```python
from build123d import *

# Parameters (mm, degrees)
SKETCH1_W                                      = 65
SKETCH1_H                                      = 40
BOSS_EXTRUDE1_DEPTH                            = 7.5
F_4_40_TAPPED_HOLE1_D                          = 2.2606
F_4_40_TAPPED_HOLE1_DEPTH                      = 7.6
F_4_40_TAPPED_HOLE1_TIP                        = 0.679152758
F_4_40_TAPPED_HOLE2_D                          = 2.2606
F_4_40_TAPPED_HOLE2_DEPTH                      = 7.6
F_4_40_TAPPED_HOLE2_TIP                        = 0.679152758
CBORE_FOR_4_SOCKET_HEAD_CAP_SCREW1_D           = 3.2639
CBORE_FOR_4_SOCKET_HEAD_CAP_SCREW1_CBORE_D     = 5.55752
CBORE_FOR_4_SOCKET_HEAD_CAP_SCREW1_CBORE_DEPTH = 2.8448


with BuildPart() as part:
    # Sketch1 → Boss-Extrude1 (new body)
    with BuildSketch(Plane(origin=(0, 0, 0), x_dir=(1, 0, 0), z_dir=(0, 1, 0))):
        Rectangle(SKETCH1_W, SKETCH1_H)
    extrude(amount=BOSS_EXTRUDE1_DEPTH)

    # #4-40 Tapped Hole1
    with Locations(Plane.XY.offset(20)):
        with Locations((-15, 3.75), (15, 3.75)):
            Hole(F_4_40_TAPPED_HOLE1_D / 2, depth=F_4_40_TAPPED_HOLE1_DEPTH)
            with Locations((0, 0, -(F_4_40_TAPPED_HOLE1_DEPTH + F_4_40_TAPPED_HOLE1_TIP / 2))):  # 118° drill point
                Cone(0, F_4_40_TAPPED_HOLE1_D / 2, F_4_40_TAPPED_HOLE1_TIP, mode=Mode.SUBTRACT)

    # #4-40 Tapped Hole2
    with Locations(Plane(origin=(0, 0, -20), x_dir=(-1, 0, 0), z_dir=(0, 0, -1))):
        with Locations((-15, 3.75), (15, 3.75)):
            Hole(F_4_40_TAPPED_HOLE2_D / 2, depth=F_4_40_TAPPED_HOLE2_DEPTH)
            with Locations((0, 0, -(F_4_40_TAPPED_HOLE2_DEPTH + F_4_40_TAPPED_HOLE2_TIP / 2))):  # 118° drill point
                Cone(0, F_4_40_TAPPED_HOLE2_D / 2, F_4_40_TAPPED_HOLE2_TIP, mode=Mode.SUBTRACT)

    # CBORE for #4 Socket Head Cap Screw1 (through all)
    with Locations(Plane(origin=(0, 0, 0), x_dir=(-1, 0, 0), z_dir=(0, -1, 0))):
        with Locations((-28.75, -10), (-28.75, 10), (28.75, 10), (28.75, -10)):
            CounterBoreHole(CBORE_FOR_4_SOCKET_HEAD_CAP_SCREW1_D / 2, CBORE_FOR_4_SOCKET_HEAD_CAP_SCREW1_CBORE_D / 2, CBORE_FOR_4_SOCKET_HEAD_CAP_SCREW1_CBORE_DEPTH)


solid = part.part
```
Read the model definition and answer for the solid it produces. Units are mm, in the model's axes. A direction names the side the tool comes from. Give positions to 0.01 mm unless a question says otherwise; leave off trailing zeros. Order: outer loops, then holes, each group sorted by start corner. A loop starts at its lowest first (then second) coordinate and runs counter-clockwise, first axis right, second up.
(1) For faces 4 (the flat face through (-31, 2.845, -10)), 5 (the cylindrical face through (14.103, 3.062, -16.147)), 6 (the cylindrical face through (-14.103, 3.062, 16.147)), determine the directions among +Z, -Z, +X, -X, +Y, -Y from which every point of the face is accessible in a straight line to the end or side of a thin tool.
(2) For a pull along X with two mould halves and no side action, classify faces 1 (the flat face through (0, 7.5, 0)), 2 (the flat face through (26.9, 2.845, 10)), 3 (the flat face through (32.5, 4, 0)) as released by +X, released by -X, zero draft, split by the parting line, or undercut.
(3) Given pin 1 (4.5 mm diameter, centred on x = 28.5, z = -10, fed in from -Y); pin 2 (1.8 mm diameter, centred on x = -15, y = 3.75, fed in from -Z), each flat-ended and moving along its own axis, determine where each tip first touches the part or whether it passes through.
(4) Find section C-C (z = -16.5). Give the vertices of the cut face in (x, y).
(5) Find section B-B (z = -10). Give the vertices of the cut face in (x, y).
(6) Straight lines are drawn through the part: L1, parallel to Z at x = 28.75, y = 4.05; L2, parallel to X at y = 5, z = -10; L3, parallel to X at y = 3.75, z = 16.75. For each, find the intervals that lie inside material, in ascending order.
(7) Find section A-A (x = -28.75). Give the vertices of the cut face in (y, z).
Result sheet:
1. face 4: -Y
1. face 5: -Z
1. face 6: +Z
2. face 1: zero draft
2. face 2: undercut
2. face 3: released by +X
3. pin 1: stops at y = 2.84
3. pin 2: stops at z = -12.26
4. outline: (-32.5, 0) - (32.5, 0) - (32.5, 7.5) - (-32.5, 7.5) - close; hole circle Ø2.26 at (-15, 3.75); hole circle Ø2.26 at (15, 3.75)
5. outline: (-32.5, 0) - (-31.53, 0) - (-31.53, 2.84) - (-30.38, 2.84) - (-30.38, 7.5) - (-32.5, 7.5) - close; (-27.12, 2.84) - (-25.97, 2.84) - (-25.97, 0) - (25.97, 0) - (25.97, 2.84) - (27.12, 2.84) - (27.12, 7.5) - (-27.12, 7.5) - close; (30.38, 2.84) - (31.53, 2.84) - (31.53, 0) - (32.5, 0) - (32.5, 7.5) - (30.38, 7.5) - close
6. L1: z = -20 to -11.63, -8.37 to 8.37, 11.63 to 20
6. L2: x = -32.5 to -30.38, -27.12 to 27.12, 30.38 to 32.5
6. L3: x = -32.5 to -16.13, -13.87 to 13.87, 16.13 to 32.5
7. outline: (0, -20) - (7.5, -20) - (7.5, -11.63) - (2.84, -11.63) - (2.84, -12.78) - (0, -12.78) - close; (0, -7.22) - (2.84, -7.22) - (2.84, -8.37) - (7.5, -8.37) - (7.5, 8.37) - (2.84, 8.37) - (2.84, 7.22) - (0, 7.22) - close; (0, 12.78) - (2.84, 12.78) - (2.84, 11.63) - (7.5, 11.63) - (7.5, 20) - (0, 20) - close
